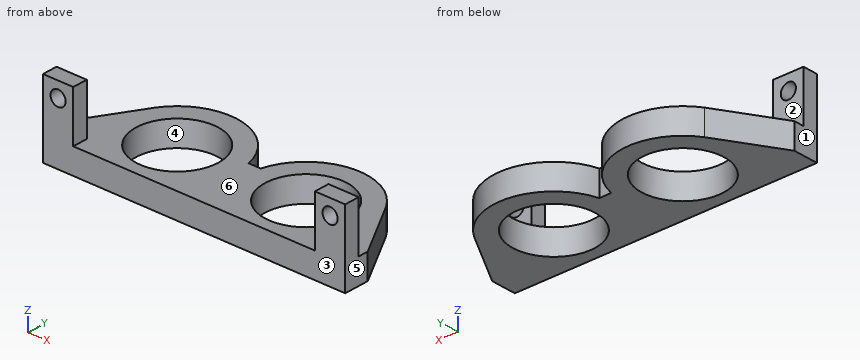
```python
from build123d import *

# Parameters (mm, degrees)
SKETCH1_R           = 8.15
BOSS_EXTRUDE1_DEPTH = 5
SKETCH3_W           = 6
SKETCH3_H           = 3
BOSS_EXTRUDE2_DEPTH = 10
SKETCH4_R           = 1.5
CUT_EXTRUDE1_DEPTH  = 10


with BuildPart() as part:
    # Sketch1 → Boss-Extrude1 (new body)
    with BuildSketch(Plane.XY):
        with BuildLine():
            Line((30, 0), (-30, 0))
            Line((-30, 0), (-30, 5))
            Line((-30, 5), (-22.877190338, 16.984968219))
            ThreePointArc((-22.877190338, 16.984968219), (-10.866798453, 22.344543701), (-1.193346785, 13.433937918))
            Line((-1.193346785, 13.433937918), (1.193346785, 13.433937918))
            ThreePointArc((1.193346785, 13.433937918), (10.866798453, 22.344543701), (22.877190338, 16.984968219))
            Line((22.877190338, 16.984968219), (30, 5))
            Line((30, 5), (30, 0))
        make_face()
        with Locations((-12.8, 10.539733165)):
            Circle(SKETCH1_R, mode=Mode.SUBTRACT)
        with Locations((12.8, 10.539733165)):
            Circle(SKETCH1_R, mode=Mode.SUBTRACT)
    extrude(amount=BOSS_EXTRUDE1_DEPTH)

    # Sketch3 → Boss-Extrude2 (add)
    with BuildSketch(Plane.XY.offset(5)):
        with Locations((-27, 1.5)):
            Rectangle(SKETCH3_W, SKETCH3_H)
        with Locations((27, 1.5)):
            Rectangle(SKETCH3_W, SKETCH3_H)
    extrude(amount=BOSS_EXTRUDE2_DEPTH)

    # Sketch4 → Cut-Extrude1 (cut)
    with BuildSketch(Plane(origin=(0, 3, 0), x_dir=(1, 0, 0), z_dir=(0, 1, 0))):
        with Locations((-27, -12)):
            Circle(SKETCH4_R)
        with Locations((27, -12)):
            Circle(SKETCH4_R)
    extrude(amount=-CUT_EXTRUDE1_DEPTH, mode=Mode.SUBTRACT)


solid = part.part
```
Model file for the job. Use its own axes, mm. Face numbers are marked on the shaded views. A direction names the side the tool comes from. Round coordinates to 2 decimals unless told otherwise and drop trailing zeros. Write each loop counter-clockwise with the first axis right and the second up, starting at its lowest first coordinate (ties: lowest second). Pieces come first, ordered by that corner, then holes. Notation, with made-up numbers: (16, 62.25) -> (24, 62.25) arc R14 cw to (24, 86.25) -> close; hole circle Ø8 at (65.25, 11.5). An arc over 180 degrees is marked (long way). Answer as CSV lines item,"result".
1. Mould opens along X. For the marked faces 3, 4, 5 and 6 say: +X half, -X half, draft (parallel to the pull), parting line (faces both ways), or undercut.
Resolved:
face 3,"draft"
face 4,"undercut"
face 5,"+X half"
face 6,"undercut"
2. Tool access for the marked faces 1 and 2: list every direction of +Z, -Z, +X, -X, +Y, -Y with a clear straight run to the whole face (end or side of a thin tool).
Resolved:
face 1,"+Z, -Z, -X, +Y, -Y"
face 2,"+Z, +X, -X, +Y"
3. Drill centre lines: line 1 (X direction, y = 1.8, z = 12); line 2 (X direction, y = 17.5, z = 4.75); line 3 (Z direction, x = -27, y = 1.5). Where is each one in solid material? Low to high.
Resolved:
line 1,"-30 to -28.5, -25.5 to -24, 24 to 25.5, 28.5 to 30"
line 2,"-22.53 to -17.04, -8.56 to -3.07, 3.07 to 8.56, 17.04 to 22.53"
line 3,"0 to 10.5, 13.5 to 15"
4. Pin check, flat tips, straight feed: pin 1 Ø1 at (x, y) = (9.5, 18.5) entering from +Z; pin 2 Ø1.2 at (x, z) = (0, 2.5) entering from +Y; pin 3 Ø5 at (x, z) = (28, 9) entering from +Y. Stop position of each tip, or through.
Resolved:
pin 1,"z = 5"
pin 2,"y = 13.43"
pin 3,"y = 3"
5. Slice it at B-B, the plane z = 5.75. List the corners of the cut face in (x, y).
Resolved:
outline,"(-30, 0) -> (-24, 0) -> (-24, 3) -> (-30, 3) -> close; (24, 0) -> (30, 0) -> (30, 3) -> (24, 3) -> close"
6. Slice it at C-C, the plane y = 12. List the corners of the cut face in (x, z).
Resolved:
outline,"(-25.84, 0) -> (-20.82, 0) -> (-20.82, 5) -> (-25.84, 5) -> close; (-4.78, 0) -> (4.78, 0) -> (4.78, 5) -> (-4.78, 5) -> close; (20.82, 0) -> (25.84, 0) -> (25.84, 5) -> (20.82, 5) -> close"
7. Slice it at D-D, the plane z = 11.25. List the corners of the cut face in (x, y).
Resolved:
outline,"(-30, 0) -> (-28.3, 0) -> (-28.3, 3) -> (-30, 3) -> close; (-25.7, 0) -> (-24, 0) -> (-24, 3) -> (-25.7, 3) -> close; (24, 0) -> (25.7, 0) -> (25.7, 3) -> (24, 3) -> close; (28.3, 0) -> (30, 0) -> (30, 3) -> (28.3, 3) -> close"
8. Slice it at A-A, the plane x = -12.8. List the corners of the cut face in (y, z).
Resolved:
outline,"(0, 0) -> (2.39, 0) -> (2.39, 5) -> (0, 5) -> close; (18.69, 0) -> (22.5, 0) -> (22.5, 5) -> (18.69, 5) -> close"
